from build123d import *

# Parameters (mm, degrees)
SKETCH1_W                   = 44.45
SKETCH1_H                   = 12.7
BOSS_EXTRUDE1_DEPTH         = 2.54
SKETCH2_W                   = 6.35
SKETCH2_H                   = 12.7
BOSS_EXTRUDE2_DEPTH         = 3.81
F_6_CLEARANCE_HOLE1_D       = 3.7973
F_3_48_TAPPED_HOLE1_D       = 1.9939
F_1_4_0_25_DIAMETER_HOLE1_D = 6.35


with BuildPart() as part:
    # Sketch1 → Boss-Extrude1 (new body)
    with BuildSketch(Plane(origin=(0, 0, 0), x_dir=(1, 0, 0), z_dir=(0, 1, 0))):
        with Locations((22.225, 6.35)):
            Rectangle(SKETCH1_W, SKETCH1_H)
    extrude(amount=BOSS_EXTRUDE1_DEPTH)

    # Sketch2 → Boss-Extrude2 (add)
    with BuildSketch(Plane.XZ):
        with Locations((3.175, -6.35)):
            Rectangle(SKETCH2_W, SKETCH2_H)
        with Locations((41.275, -6.35)):
            Rectangle(SKETCH2_W, SKETCH2_H)
    extrude(amount=BOSS_EXTRUDE2_DEPTH)

    # #6 Clearance Hole1 (through all)
    with Locations(Plane(origin=(0, 2.54, 0), x_dir=(1, 0, 0), z_dir=(0, 1, 0))):
        with Locations((3.175, 6.35), (41.275, 6.35)):
            Hole(F_6_CLEARANCE_HOLE1_D / 2)

    # #3-48 Tapped Hole1 (through all)
    with Locations(Plane(origin=(0, 2.54, 0), x_dir=(1, 0, 0), z_dir=(0, 1, 0))):
        with Locations((14.7828, 6.35), (29.6672, 6.35)):
            Hole(F_3_48_TAPPED_HOLE1_D / 2)

    # 1/4 (0.25) Diameter Hole1 (through all)
    with Locations(Plane(origin=(0, 2.54, 0), x_dir=(1, 0, 0), z_dir=(0, 1, 0))):
        with Locations((22.225, 6.35)):
            Hole(F_1_4_0_25_DIAMETER_HOLE1_D / 2)


solid = part.part
Design review of the part built by this model. Coordinates are the model's own, in mm. A direction names the side the tool comes from. Round coordinates to 2 decimals unless told otherwise and drop trailing zeros. Write each loop counter-clockwise with the first axis right and the second up, starting at its lowest first coordinate (ties: lowest second). Pieces come first, ordered by that corner, then holes.
Item 1: Draft analysis for pull direction X (two halves, no side actions). For faces 1 (the flat face through (44.45, -1, -6)), 2 (the flat face through (6.35, -2, -6)), 3 (the flat face through (22, 1, -12.7)), state which applies: released by +X, released by -X, zero draft, split by the parting line, or undercut.
Item 2: Consider section C-C on x = 4. Give the boundary of the cut face in (y, z).
Item 3: For faces 4 (the flat face through (0, -1, -6)), 5 (the flat face through (38.1, -2, -6)), list the 3-axis set-ups (+Z, -Z, +X, -X, +Y, -Y) from which the entire face can be reached by the end or side of a thin tool; tool diameter is ignored.
Item 4: Consider section A-A on y = -1. Give the boundary of the cut face in (x, z) (3 decimals), and give its area (3 significant figures).
Item 5: Consider section B-B on z = -6.35. Give the boundary of the cut face in (x, y).
Item 6: For pin 1 Ø1 at (x, z) = (15, -8) entering from -Y; pin 2 Ø1.2 at (x, z) = (29.67, -6.35) entering from -Y, all flat-tipped, find the tip position at first contact; note any pin that passes through.
Item 7: Consider section D-D on y = 1.5. Give the boundary of the cut face in (x, z) (3 decimals), and give its area (3 significant figures).
Item 8: Wall thickness on L1, parallel to X at y = -2.75, z = -9; L2, parallel to Y at x = 17.5, z = -4; L3, parallel to X at y = 0.25, z = -9: over which ranges is each line inside the solid? List them lowest first.
Check values:
1. face 1: released by +X
1. face 2: undercut
1. face 3: zero draft
2. outline: (-3.81, -12.7) - (2.54, -12.7) - (2.54, -8.06) - (-3.81, -8.06) - close; (-3.81, -4.64) - (2.54, -4.64) - (2.54, 0) - (-3.81, 0) - close
3. face 4: +Z, -Z, -X, +Y, -Y
3. face 5: +Z, -Z, -Y
4. outline: (0, -12.7) - (6.35, -12.7) - (6.35, 0) - (0, 0) - close; (38.1, -12.7) - (44.45, -12.7) - (44.45, 0) - (38.1, 0) - close; hole circle Ø3.797 at (3.175, -6.35); hole circle Ø3.797 at (41.275, -6.35)
4. area: 139 mm2
5. outline: (0, -3.81) - (1.28, -3.81) - (1.28, 2.54) - (0, 2.54) - close; (5.07, -3.81) - (6.35, -3.81) - (6.35, 0) - (13.79, 0) - (13.79, 2.54) - (5.07, 2.54) - close; (15.78, 0) - (19.05, 0) - (19.05, 2.54) - (15.78, 2.54) - close; (25.4, 0) - (28.67, 0) - (28.67, 2.54) - (25.4, 2.54) - close; (30.66, 0) - (38.1, 0) - (38.1, -3.81) - (39.38, -3.81) - (39.38, 2.54) - (30.66, 2.54) - close; (43.17, -3.81) - (44.45, -3.81) - (44.45, 2.54) - (43.17, 2.54) - close
6. pin 1: stops at y = 0
6. pin 2: passes through
7. outline: (0, -12.7) - (44.45, -12.7) - (44.45, 0) - (0, 0) - close; hole circle Ø3.797 at (3.175, -6.35); hole circle Ø1.994 at (14.783, -6.35); hole circle Ø6.35 at (22.225, -6.35); hole circle Ø1.994 at (29.667, -6.35); hole circle Ø3.797 at (41.275, -6.35)
7. area: 504 mm2
8. L1: x = 0 to 6.35, 38.1 to 44.45
8. L2: y = 0 to 2.54
8. L3: x = 0 to 20.48, 23.97 to 44.45
